from build123d import *

# Parameters (mm, degrees)
SKETCH1_W           = 10.16
SKETCH1_H           = 7.62
SKETCH1_R           = 2.2225
BOSS_EXTRUDE1_DEPTH = 2.54
SKETCH1_4_W         = 10.16
SKETCH1_4_H         = 2.54
BOSS_EXTRUDE2_DEPTH = 20.32
FILLET1_R           = 2.54
CUT_EXTRUDE1_REACH  = 24.288
SKETCH2_R           = 2.2225


with BuildPart() as part:
    # Sketch1 → Boss-Extrude1 (new body)
    with BuildSketch(Plane(origin=(0, 0, 0), x_dir=(1, 0, 0), z_dir=(0, 1, 0))):
        with Locations((0, -1.27)):
            Rectangle(SKETCH1_W, SKETCH1_H)
        with Locations(Location((0, 0, 0), (0, 0, 270))):
            Circle(SKETCH1_R, mode=Mode.SUBTRACT)
    extrude(amount=BOSS_EXTRUDE1_DEPTH)

    # Sketch1_4 → Boss-Extrude2 (add)
    with BuildSketch(Plane(origin=(0, 0, 0), x_dir=(1, 0, 0), z_dir=(0, 1, 0))):
        with Locations((0, 3.81)):
            Rectangle(SKETCH1_4_W, SKETCH1_4_H)
    extrude(amount=BOSS_EXTRUDE2_DEPTH)

    # Fillet1
    fillet1_edges = [part.edges().sort_by_distance(p)[0] for p in [
        (0, 0, -5.08),
    ]]
    fillet(fillet1_edges, radius=FILLET1_R)

    # Sketch2 → Cut-Extrude1 (cut, up to next)
    with BuildSketch(Plane.XY.offset(-2.54), mode=Mode.PRIVATE) as cut_extrude1_sk1:
        with Locations((0, 15.3416)):
            Circle(SKETCH2_R)
    cut_extrude1_tool1 = extrude(cut_extrude1_sk1.sketch, amount=-CUT_EXTRUDE1_REACH, mode=Mode.PRIVATE) & part.part
    add(cut_extrude1_tool1.solids().sort_by_distance((0, 15.3416, -2.54))[0], mode=Mode.SUBTRACT)


solid = part.part
Geometry: final body of the model. Coordinates: model frame, mm. A direction names the side the tool comes from. Give positions to 0.01 mm unless a question says otherwise; leave off trailing zeros. Order: outer loops, then holes, each group sorted by start corner. A loop starts at its lowest first (then second) coordinate and runs counter-clockwise, first axis right, second up. Notation, with made-up numbers: (39.25, -31) -> (54.25, -31) arc R24 cw to (54.25, -5) -> close; hole circle Ø9 at (60.25, 57). An arc over 180 degrees is marked (long way). Put each result on its own line as item: value.
Q1. Section D-D, the plane y = 19. Return loops of the section in (x, z), then the cut area to 3 significant figures.
Here are the results:
outline: (-5.08, -5.08) -> (5.08, -5.08) -> (5.08, -2.54) -> (-5.08, -2.54) -> close
area: 25.8 mm^2
Q2. Section C-C, the plane x = -2.5. Return loops of the section in (y, z), then the cut area to 3 significant figures.
Here are the results:
outline: (0, -2.54) arc R2.54 ccw to (2.54, -5.08) -> (20.32, -5.08) -> (20.32, -2.54) -> (2.54, -2.54) -> (2.54, 5.08) -> (0, 5.08) -> close
area: 69.6 mm^2
Q3. Pin query (flat end, axial travel): pin 1 (1.5 mm diameter, centred on y = 14, z = -2.5, fed in from +X); pin 2 (5 mm diameter, centred on x = -2, y = 7, fed in from +Z). Return the tip coordinate at first contact, or that it passes through.
Here are the results:
pin 1: stops at x = 5.08
pin 2: stops at z = -2.54
Q4. Material intervals for L1, parallel to X at y = 1, z = 0; L2, parallel to Z at x = 0.5, y = 7.25; L3, parallel to Y at x = 0, z = -4, sorted ascending.
Here are the results:
L1: x = -5.08 to -2.22, 2.22 to 5.08
L2: z = -5.08 to -2.54
L3: y = 0.46 to 13.12, 17.56 to 20.32
Q5. Draft query along X for faces 1 (the face through (-5.08, 8, -3)), 2 (the face through (0, 11, -5.08)), 3 (the face through (-0.289, 17.545, -3.792)). Return one class per face: released by +X, released by -X, zero draft, split by the parting line, or undercut.
Here are the results:
face 1: released by -X
face 2: zero draft
face 3: undercut
Q6. Section A-A, the plane z = 0. Return loops of the section in (x, y), then the cut area to 3 significant figures.
Here are the results:
outline: (-5.08, 0) -> (-2.22, 0) -> (-2.22, 2.54) -> (-5.08, 2.54) -> close; (2.22, 0) -> (5.08, 0) -> (5.08, 2.54) -> (2.22, 2.54) -> close
area: 14.5 mm^2
Q7. Reachability of faces 4 (the face through (-1.2, 2.54, 2.1)), 5 (the face through (0, 20.32, -4)) from +Z, -Z, +X, -X, +Y, -Y: full face, straight path, thin tool, end or side. Return the list, or none.
Here are the results:
face 4: +Z, +X, -X, +Y
face 5: +Z, -Z, +X, -X, +Y
Q8. Section B-B, the plane x = 0. Return loops of the section in (y, z), then the cut area to 3 significant figures.
Here are the results:
outline: (0, -2.54) arc R2.54 ccw to (2.54, -5.08) -> (13.12, -5.08) -> (13.12, -2.54) -> (2.54, -2.54) -> (2.54, -2.22) -> (0, -2.22) -> close; (0, 2.22) -> (2.54, 2.22) -> (2.54, 5.08) -> (0, 5.08) -> close; (17.56, -5.08) -> (20.32, -5.08) -> (20.32, -2.54) -> (17.56, -2.54) -> close
area: 47.0 mm^2
